```python
from build123d import *

# Parameters (mm, degrees)
MODEL_R                 = 1.5
SALIENTE_EXTRUIR1_DEPTH = 3


with BuildPart() as part:
    # Model → Saliente-Extruir1 (new body)
    with BuildSketch(Plane.XY):
        with BuildLine():
            Line((174.227054575, 213.178720063), (174.227054575, 204.178720063))
            ThreePointArc((174.227054575, 204.178720063), (174.569596678, 202.456644617), (175.545074059, 200.996739548))
            Line((175.545074059, 200.996739548), (184.545074059, 191.996739548))
            ThreePointArc((184.545074059, 191.996739548), (187.727054575, 190.678720063), (190.90903509, 191.996739548))
            Line((190.90903509, 191.996739548), (199.90903509, 200.996739548))
            ThreePointArc((199.90903509, 200.996739548), (200.884512471, 202.456644617), (201.227054575, 204.178720063))
            Line((201.227054575, 204.178720063), (201.227054575, 222.178720063))
            ThreePointArc((201.227054575, 222.178720063), (199.90903509, 225.360700578), (196.727054575, 226.678720063))
            Line((196.727054575, 226.678720063), (178.727054575, 226.678720063))
            ThreePointArc((178.727054575, 226.678720063), (175.545074059, 225.360700578), (174.227054575, 222.178720063))
            Line((174.227054575, 222.178720063), (174.227054575, 213.178720063))
        make_face()
        with Locations((187.727054575, 204.178720063)):
            Circle(MODEL_R, mode=Mode.SUBTRACT)
        with Locations((178.727054575, 204.178720063)):
            Circle(MODEL_R, mode=Mode.SUBTRACT)
        with Locations((187.727054575, 213.178720063)):
            Circle(MODEL_R, mode=Mode.SUBTRACT)
        with Locations((178.727054575, 213.178720063)):
            Circle(MODEL_R, mode=Mode.SUBTRACT)
        with Locations((196.727054575, 213.178720063)):
            Circle(MODEL_R, mode=Mode.SUBTRACT)
        with Locations((187.727054575, 195.178720063)):
            Circle(MODEL_R, mode=Mode.SUBTRACT)
        with Locations((196.727054575, 204.178720063)):
            Circle(MODEL_R, mode=Mode.SUBTRACT)
        with Locations((187.727054575, 222.178720063)):
            Circle(MODEL_R, mode=Mode.SUBTRACT)
        with Locations((178.727054575, 222.178720063)):
            Circle(MODEL_R, mode=Mode.SUBTRACT)
        with Locations((196.727054575, 222.178720063)):
            Circle(MODEL_R, mode=Mode.SUBTRACT)
    extrude(amount=SALIENTE_EXTRUIR1_DEPTH)


solid = part.part
```
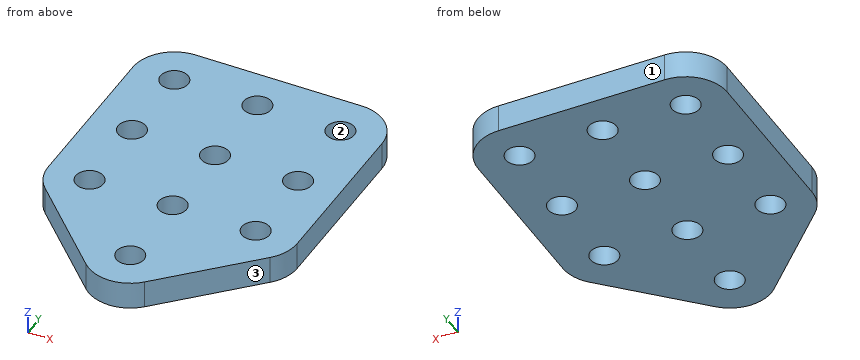
Verification items for the finished model (mm, model axes). Face numbers are marked on the shaded views. Give positions to 0.01 mm unless a question says otherwise; leave off trailing zeros. Order: outer loops, then holes, each group sorted by start corner. A loop starts at its lowest first (then second) coordinate and runs counter-clockwise, first axis right, second up. Notation, with made-up numbers: (76, 77.25) - (133, 77.25) arc R34 cw to (133, 111.25) - close; hole circle Ø8 at (6.25, 51.5). An arc over 180 degrees is marked (long way). Answer as CSV lines item,"result". Start each with the question number.
Item 1: Mould release check, pull along Y, two halves, no side actions. Record for the marked faces 1, 2 and 3: released by +Y, released by -Y, zero draft, split by the parting line, or undercut.
Item 2: Material ranges on L1, parallel to Y at x = 179, z = 2.4; L2, parallel to X at y = 203, z = 1.25; L3, parallel to Y at x = 178.5, z = 1.9, recorded low to high.
Item 3: Section check B-B, the plane y = 196. Record the boundary of the cut face in (x, z).
Item 4: Section check C-C, the plane z = 1.2. State how many separate pieces and enclosed holes the cut face has, plus the area to 3 significant figures.
Item 5: Section check D-D, the plane y = 221.5. Record the boundary of the cut face in (x, z), plus the area to 3 significant figures.
Item 6: Section check A-A, the plane x = 179.75. Record the boundary of the cut face in (y, z), plus the area to 3 significant figures.
Filled in:
1,face 1,"released by +Y"
1,face 2,"undercut"
1,face 3,"released by -Y"
2,L1,"197.54 to 202.7, 205.65 to 211.7, 214.65 to 220.7, 223.65 to 226.68"
2,L2,"174.38 to 177.8, 179.65 to 186.8, 188.65 to 195.8, 197.65 to 201.07"
2,L3,"198.04 to 202.7, 205.66 to 211.7, 214.66 to 220.7, 223.66 to 226.67"
3,outline,"(180.54, 0) - (186.47, 0) - (186.47, 3) - (180.54, 3) - close; (188.98, 0) - (194.91, 0) - (194.91, 3) - (188.98, 3) - close"
4,separate pieces,"1"
4,enclosed holes,"10"
4,area,"755 mm^2"
5,outline,"(174.23, 0) - (177.39, 0) - (177.39, 3) - (174.23, 3) - close; (180.06, 0) - (186.39, 0) - (186.39, 3) - (180.06, 3) - close; (189.06, 0) - (195.39, 0) - (195.39, 3) - (189.06, 3) - close; (198.06, 0) - (201.23, 0) - (201.23, 3) - (198.06, 3) - close"
5,area,"56.9 mm^2"
6,outline,"(196.79, 0) - (203.08, 0) - (203.08, 3) - (196.79, 3) - close; (205.28, 0) - (212.08, 0) - (212.08, 3) - (205.28, 3) - close; (214.28, 0) - (221.08, 0) - (221.08, 3) - (214.28, 3) - close; (223.28, 0) - (226.68, 0) - (226.68, 3) - (223.28, 3) - close"
6,area,"69.9 mm^2"
